The figure shows three views and two pictorial views of one solid part (mm, origin at its lowest corner). Answer the questions. A direction names the side the tool comes from. Round coordinates to 2 decimals unless told otherwise and drop trailing zeros. Order: outer loops, then holes, each group sorted by start corner. A loop starts at its lowest first (then second) coordinate and runs counter-clockwise, first axis right, second up. Notation, with made-up numbers: (13, 48) - (53, 48) arc R12 ccw to (53, 55) - close; hole circle Ø6 at (30.25, 47). An arc over 180 degrees is marked (long way). Answer in a Markdown table with one row per item.
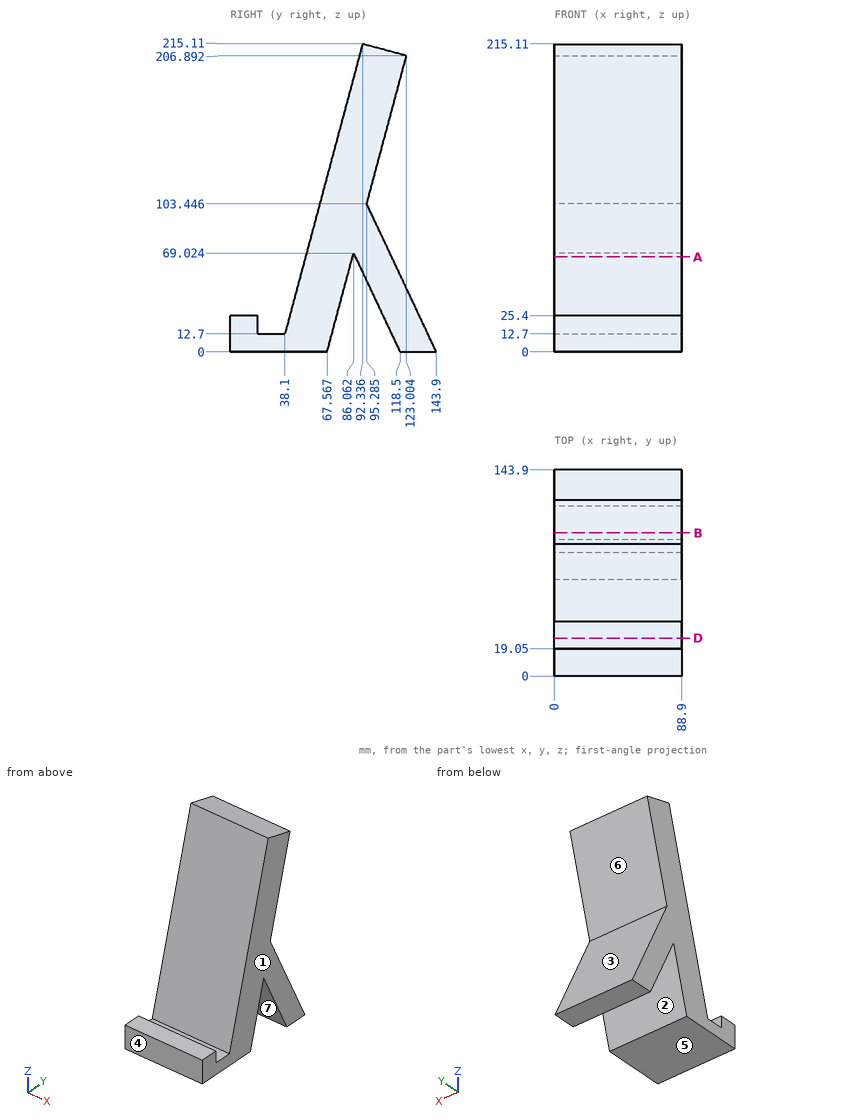
1) The mould has two halves that part along Y. Classify the marked faces 1, 2, 3 and 4: released by +Y, released by -Y, zero draft, split by the parting line, or undercut.
Filled in:
| item | result |
|---|---|
| face 1 | zero draft |
| face 2 | undercut |
| face 3 | released by +Y |
| face 4 | released by -Y |
2) Which of the six approach directions +Z, -Z, +X, -X, +Y, -Y give full straight-line access (tool end or side, diameter ignored) to the marked faces 5, 6 and 7?
Filled in:
| item | result |
|---|---|
| face 5 | -Z, +X, -X, +Y, -Y |
| face 6 | +X, -X, +Y |
| face 7 | -Z, +X, -X |
3) Find the intervals of material crossed by probe 1 along Y at (x, z) = (82, 23); probe 2 along Z at (x, y) = (23.5, 30.5); probe 3 along Y at (x, z) = (16, 26) (1 decimal), in increasing order. Write a range as from..to.
Filled in:
| item | result |
|---|---|
| probe 1 | y = 0..19.05, 40.86..73.73, 107.69..133.09 |
| probe 2 | z = 0..12.7 |
| probe 3 | y = 41.7..74.5, 106.3..131.7 |
4) Find section D-D, the plane y = 26.5. Give the vertices of the cut face in (x, z).
Filled in:
| item | result |
|---|---|
| outline | (0, 0) - (88.9, 0) - (88.9, 12.7) - (0, 12.7) - close |
5) Find section A-A, the plane z = 66.5. Give the vertices of the cut face in (x, y) (1 decimal).
Filled in:
| item | result |
|---|---|
| outline | (0, 52.5) - (88.9, 52.5) - (88.9, 85.4) - (0, 85.4) - close; (0, 87.2) - (88.9, 87.2) - (88.9, 112.6) - (0, 112.6) - close |
6) Each of these flat-tipped pins is pushed along its axis until it touches: pin 1 (5.5 mm diameter, centred on x = 48.5, y = 12.5, fed in from +Z); pin 2 (6 mm diameter, centred on x = 80, z = 167.5, fed in from +Y); pin 3 (4 mm diameter, centred on x = 33.5, z = 148, fed in from -Y). Where does it stop, or does it pass through?
Filled in:
| item | result |
|---|---|
| pin 1 | stops at z = 25.4 |
| pin 2 | stops at y = 113.25 |
| pin 3 | stops at y = 73.82 |
7) Find section B-B, the plane y = 100. Give the vertices of the cut face in (x, z) (1 decimal), then the cut area to 3 significant figures.
Filled in:
| item | result |
|---|---|
| outline | (0, 39.4) - (88.9, 39.4) - (88.9, 93.4) - (0, 93.4) - close; (0, 121) - (88.9, 121) - (88.9, 213.1) - (0, 213.1) - close |
| area | 13,000 mm^2 |
